from build123d import *

# Parameters (mm, degrees)
BOSS_EXTRUDE1_DEPTH = 5
CUT_EXTRUDE3_DEPTH  = 3
FILLET2_R           = 10
FILLET3_R           = 5
FILLET4_R           = 2


with BuildPart() as part:
    # Sketch1 → Boss-Extrude1 (new body)
    with BuildSketch(Plane(origin=(0, 0, 0), x_dir=(1, 0, 0), z_dir=(0, 1, 0))):
        Polygon((0, 4), (13, 4), (13, 46.73), (11, 46.73), (11, 52.1), (13, 52.1), (13, 56), (21, 56), (21, 52.1), (23, 52.1), (23, 46.73), (21, 46.73), (21, 4), (21, -4), (13, -4), (0, -4), (-8, -4), (-8, 14), (0, 14), align=None)
    extrude(amount=BOSS_EXTRUDE1_DEPTH)

    # Sketch2 → Cut-Extrude3 (cut)
    with BuildSketch(Plane(origin=(0, 5, 0), x_dir=(1, 0, 0), z_dir=(0, 1, 0))):
        with BuildLine():
            Line((19.921, 46.641739258), (18.923587356, 34.436800493))
            ThreePointArc((18.923587356, 34.436800493), (17, 32.664), (15.076412644, 34.436800493))
            Line((15.076412644, 34.436800493), (14.079, 46.641739258))
            ThreePointArc((14.079, 46.641739258), (17, 52.4), (19.921, 46.641739258))
        make_face()
    extrude(amount=-CUT_EXTRUDE3_DEPTH, mode=Mode.SUBTRACT)

    # Fillet2
    fillet2_edges = [part.edges().sort_by_distance(p)[0] for p in [
        (21, 2.5, 4),
        (-8, 2.5, 4),
    ]]
    fillet(fillet2_edges, radius=FILLET2_R)

    # Fillet3
    # the kernel refuses this fillet: 5 mm, written as the material it takes off along each edge
    with BuildSketch(Plane(origin=(0, -12.5, -14), x_dir=(-1, 0, 0), z_dir=(0, 1, 0)), Plane(origin=(-8, -12.5, -14), x_dir=(0, 0, 1), z_dir=(0, 1, 0))) as fillet3_piece_1:
        with BuildLine():
            CenterArc((FILLET3_R, FILLET3_R), FILLET3_R, 180, 90)
            Line((0, FILLET3_R), (0, 0))
            Line((0, 0), (FILLET3_R, 0))
        make_face()
    extrude(amount=30, mode=Mode.SUBTRACT)

    # Fillet4
    fillet4_edges = [part.edges().sort_by_distance(p)[0] for p in [
        (0, 2.5, -4),
        (13, 2.5, -4),
    ]]
    fillet(fillet4_edges, radius=FILLET4_R)


solid = part.part
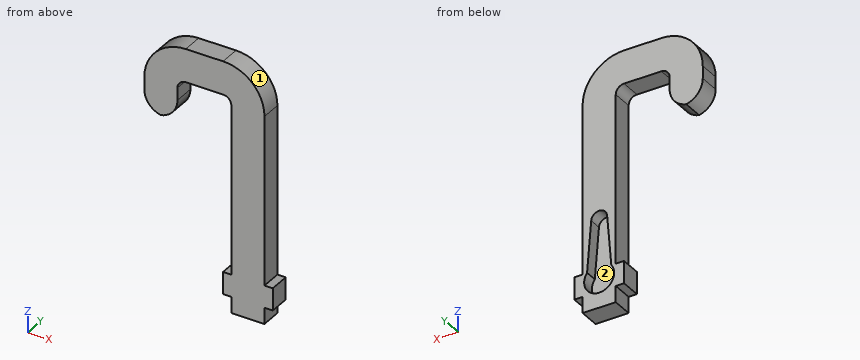
Model file for the job. Use its own axes, mm. Face numbers are marked on the shaded views. A direction names the side the tool comes from. Give positions to 0.01 mm unless a question says otherwise; leave off trailing zeros. Loops run counter-clockwise (first coordinate to the right, second up) from the corner with the lowest first, then second, coordinate; pieces in that order, holes last. Notation, with made-up numbers: (-23, 87.5) -> (14, 87.5) arc R23 ccw to (14, 105.5) -> close; hole circle Ø9 at (52.25, 74). An arc over 180 degrees is marked (long way). Use a Markdown table: item, result. Add a question column.
(1) Slice it at C-C on x = 17. List the corners of the cut face in (y, z), and give its area (3 significant figures).
(2) Slice it at D-D on y = 0.7. List the corners of the cut face in (x, z), and give its area (3 significant figures).
(3) Slice it at B-B on z = -48.78. List the corners of the cut face in (x, y), and give its area (3 significant figures).
(4) Drop flat-ended pins along their axis: pin 1 Ø2.5 at (y, z) = (1.5, -23) entering from -X; pin 2 Ø1.5 at (y, z) = (1.5, -32.5) entering from +X; pin 3 Ø0.6 at (x, y) = (12.5, 2) entering from -Z. Give the stop position or say it passes through.
(5) Wall check: line 1 along Z through (x, y) = (17, 4.4); line 2 along X through (y, z) = (2.9, -48.78); line 3 along X through (y, z) = (3.8, -6.5). Give the ranges that are in metal, low to high.
(6) Slice it at A-A on y = 3.35. List the corners of the cut face in (x, z), and give its area (3 significant figures).
(7) Tool access for the marked faces 1 and 2: list every direction of +Z, -Z, +X, -X, +Y, -Y with a clear straight run to the whole face (end or side of a thin tool).
Filled sheet:
| question | item | result |
|---|---|---|
| 1 | outline | (0, -56) -> (5, -56) -> (5, -52.4) -> (2, -52.4) -> (2, -32.66) -> (5, -32.66) -> (5, 2) -> (0, 2) -> close |
| 1 | area | 231 mm2 |
| 2 | outline | (-8, -9) arc R5 ccw to (-4, -13.9) arc R5 ccw to (0, -9) -> (0, -6) arc R2 cw to (2, -4) -> (11, -4) arc R2 cw to (13, -6) -> (13, -46.73) -> (11, -46.73) -> (11, -52.1) -> (13, -52.1) -> (13, -56) -> (21, -56) -> (21, -52.1) -> (23, -52.1) -> (23, -46.73) -> (21, -46.73) -> (21, -6) arc R10 ccw to (11, 4) -> (2, 4) arc R10 ccw to (-8, -6) -> close |
| 2 | area | 698 mm2 |
| 3 | outline | (11, 0) -> (23, 0) -> (23, 5) -> (20.62, 5) -> (20.62, 2) -> (13.38, 2) -> (13.38, 5) -> (11, 5) -> close |
| 3 | area | 38.3 mm2 |
| 4 | pin 1 | x = 13 |
| 4 | pin 2 | x = 21 |
| 4 | pin 3 | z = -52.1 |
| 5 | line 1 | -56 to -52.4, -32.66 to 2 |
| 5 | line 2 | 11 to 13.38, 20.62 to 23 |
| 5 | line 3 | -8 to 0, 13 to 21 |
| 6 | outline | (-8, -9) arc R5 ccw to (-4, -13.9) arc R5 ccw to (0, -9) -> (0, -6) arc R2 cw to (2, -4) -> (11, -4) arc R2 cw to (13, -6) -> (13, -46.73) -> (11, -46.73) -> (11, -52.1) -> (13, -52.1) -> (13, -56) -> (21, -56) -> (21, -52.1) -> (23, -52.1) -> (23, -46.73) -> (21, -46.73) -> (21, -6) arc R10 ccw to (11, 4) -> (2, 4) arc R10 ccw to (-8, -6) -> close; hole (14.08, -46.64) arc R3.62 ccw (long way) to (19.92, -46.64) -> (18.92, -34.44) arc R1.93 ccw to (15.08, -34.44) -> close |
| 6 | area | 598 mm2 |
| 7 | face 1 | +Z, +X, +Y, -Y |
| 7 | face 2 | +Y |
